from build123d import *

# Parameters (mm, degrees)
F1_DEPTH = 2.5
F3_DEPTH = 2
F4_R     = 0.87499
F6_DEPTH = 4
F7_R     = 0.75


# Not quite as in the source:
# - a fillet or chamfer is up to 0.001 mm smaller than in the source, because OpenCascade refuses the exact size


with BuildPart() as f1:
    # F0 (on Top) → F1 (new body)
    with BuildSketch(Plane.XY):
        with BuildLine():
            Line((-5, -10), (5, -10))
            ThreePointArc((5, -10), (8.5355339059, -8.5355339059), (10, -5))
            Line((10, -5), (10, 5))
            ThreePointArc((10, 5), (8.5355339059, 8.5355339059), (5, 10))
            Line((5, 10), (-5, 10))
            ThreePointArc((-5, 10), (-8.5355339059, 8.5355339059), (-10, 5))
            Line((-10, 5), (-10, -5))
            ThreePointArc((-10, -5), (-8.5355339059, -8.5355339059), (-5, -10))
        make_face()
    extrude(amount=F1_DEPTH)

    # F2 (on face) → F3 (join)
    with BuildSketch(Plane.XY.offset(2.5)):
        with BuildLine():
            Line((-5, -11.5), (5, -11.5))
            ThreePointArc((5, -11.5), (9.5961940777, -9.5961940777), (11.5, -5))
            Line((11.5, -5), (11.5, 5))
            ThreePointArc((11.5, 5), (9.5961940777, 9.5961940777), (5, 11.5))
            Line((5, 11.5), (-5, 11.5))
            ThreePointArc((-5, 11.5), (-9.5961940777, 9.5961940777), (-11.5, 5))
            Line((-11.5, 5), (-11.5, -5))
            ThreePointArc((-11.5, -5), (-9.5961940777, -9.5961940777), (-5, -11.5))
        make_face()
        with BuildLine():
            ThreePointArc((9.75, -5), (8.3587572106, -8.3587572106), (5, -9.75))
            Line((5, -9.75), (-5, -9.75))
            ThreePointArc((-5, -9.75), (-8.3587572106, -8.3587572106), (-9.75, -5))
            Line((-9.75, -5), (-9.75, 5))
            ThreePointArc((-9.75, 5), (-8.3587572106, 8.3587572106), (-5, 9.75))
            Line((-5, 9.75), (5, 9.75))
            ThreePointArc((5, 9.75), (8.3587572106, 8.3587572106), (9.75, 5))
            Line((9.75, 5), (9.75, -5))
        make_face(mode=Mode.SUBTRACT)
    extrude(amount=F3_DEPTH)

    # F4 (radius 0.875 in the source; OpenCascade refuses exactly that, so slightly less here)
    f4_edges = [f1.edges().sort_by_distance(p)[0] for p in [
        (-9.75, 0, 4.5),
        (-11.5, 0, 4.5),
    ]]
    fillet(f4_edges, radius=F4_R)

    # F5 (on face) → F6 (join)
    with BuildSketch(Plane.XY.offset(2.5)):
        with BuildLine():
            ThreePointArc((9.5, 5), (8.1819805153, 8.1819805153), (5, 9.5))
            Line((5, 9.5), (-5, 9.5))
            ThreePointArc((-5, 9.5), (-8.1819805153, 8.1819805153), (-9.5, 5))
            Line((-9.5, 5), (-9.5, -5))
            ThreePointArc((-9.5, -5), (-8.1819805153, -8.1819805153), (-5, -9.5))
            Line((-5, -9.5), (5, -9.5))
            ThreePointArc((5, -9.5), (8.1819805153, -8.1819805153), (9.5, -5))
            Line((9.5, -5), (9.5, 5))
        make_face()
    extrude(amount=F6_DEPTH)

    # F7
    f7_edges = [f1.edges().sort_by_distance(p)[0] for p in [
        (0, -9.5, 6.5),
    ]]
    fillet(f7_edges, radius=F7_R)


solid = f1.part
Verification items for the finished model (mm, model axes). A direction names the side the tool comes from. Round coordinates to 2 decimals unless told otherwise and drop trailing zeros. Write each loop counter-clockwise with the first axis right and the second up, starting at its lowest first coordinate (ties: lowest second). Pieces come first, ordered by that corner, then holes.
(1) Depth check by flat-ended pin: pin 1 Ø0.8 at (y, z) = (0, 1.5) entering from -X; pin 2 Ø1.2 at (x, z) = (2, 1.5) entering from -Y; pin 3 Ø1.5 at (x, z) = (8.5, 3) entering from +Y. Enter the tip coordinate at first touch or a pass-through.
Returned:
pin 1: stops at x = -10
pin 2: stops at y = -10
pin 3: stops at y = 10.89
(2) Section check D-D (z = 1.25). Enter the section's corners in (x, y).
Returned:
outline: (-10, -5) arc R5 ccw to (-5, -10) - (5, -10) arc R5 ccw to (10, -5) - (10, 5) arc R5 ccw to (5, 10) - (-5, 10) arc R5 ccw to (-10, 5) - close
(3) Material ranges on line 1 (Y direction, x = -1, z = 3); line 2 (X direction, y = -7.5, z = 4.25), recorded low to high.
Returned:
line 1: y = -11.5 to -9.75, -9.5 to 9.5, 9.75 to 11.5
line 2: x = -10.71 to -9.34, -8.74 to 8.74, 9.34 to 10.71
(4) Access from +Z, -Z, +X, -X, +Y, -Y to the whole of each face (thin tool, end or side, straight path). Record for faces 1 (the flat face through (-10, 0, 1)), 2 (the flat face through (9.5, 0, 4)), 3 (the flat face through (-0.1, -10.2, 2.5)).
Returned:
face 1: -Z, -X, +Y, -Y
face 2: +Z
face 3: -Z
(5) Mould release check, pull along Y, two halves, no side actions. Record for faces 4 (the flat face through (0, 10, 1)), 5 (the cylindrical face through (8.322, 8.395, 3.055)), 6 (the flat face through (0, 0, 0)): pulls with the +Y half, pulls with the -Y half, needs draft (parallel to the pull), parting line crosses it, or undercut.
Returned:
face 4: pulls with the +Y half
face 5: undercut
face 6: needs draft
(6) Section check A-A (z = 5). Enter the section's corners in (x, y).
Returned:
outline: (-9.5, -5) arc R4.5 ccw to (-5, -9.5) - (5, -9.5) arc R4.5 ccw to (9.5, -5) - (9.5, 5) arc R4.5 ccw to (5, 9.5) - (-5, 9.5) arc R4.5 ccw to (-9.5, 5) - close
